The listing builds one solid part. Answer for the finished solid, in the listing's coordinates (mm). A direction names the side the tool comes from. Round coordinates to 2 decimals unless told otherwise and drop trailing zeros. Write each loop counter-clockwise with the first axis right and the second up, starting at its lowest first coordinate (ties: lowest second). Pieces come first, ordered by that corner, then holes.
Item 1: Find section B-B on x = 5. Give the vertices of the cut face in (y, z).
Item 2: Find section A-A on z = 5. Give the vertices of the cut face in (x, y), then the cut area to 3 significant figures.
Item 3: Find section D-D on z = 70. Give the vertices of the cut face in (x, y), then the cut area to 3 significant figures.
Item 4: A tool of negligible diameter and unlimited length cuts with its end or side. For faces 4 (the face through (0.5, 5.1, 80)), 5 (the face through (1, 5, 41)), from which of +Z, -Z, +X, -X, +Y, -Y can it reach the whole face along a straight path? Write none if from no direction.
Item 5: For a pull along Z with two mould halves and no side action, classify faces 1 (the face through (10, 5, 41)), 2 (the face through (9.507, 5.481, 76.526)), 3 (the face through (0.5, 5.1, 0)) as +Z half, -Z half, draft (parallel to the pull), parting line (faces both ways), or undercut.
Item 6: Find the intervals of material crossed by probe 1 along Z at (x, y) = (5, 0.35); probe 2 along X at (y, z) = (5.75, 23.5); probe 3 along X at (y, z) = (0.7, 15), in increasing order.
Item 7: Find section C-C on y = 2.5. Give the vertices of the cut face in (x, z), then the cut area to 3 significant figures.
```python
from build123d import *

# Parameters (mm, degrees)
SKETCH_1_W          = 10
SKETCH_1_H          = 10
SKETCH_1_W_2        = 8
SKETCH_1_H_2        = 8
EXTRUDE_1_DEPTH     = 40
SKETCH_2_R          = 1.6
CUT_EXTRUDE_1_DEPTH = 11
SKETCH_3_R          = 1.6
CUT_EXTRUDE_2_DEPTH = 11


with BuildPart() as part:
    # ｽｹｯﾁ1 → ﾎﾞｽ - 押し出し1 (new body)
    with BuildSketch(Plane.XY):
        with Locations((5, 5)):
            Rectangle(SKETCH_1_W, SKETCH_1_H)
        with Locations((5, 5)):
            Rectangle(SKETCH_1_W_2, SKETCH_1_H_2, mode=Mode.SUBTRACT)
    extrude(amount=EXTRUDE_1_DEPTH)

    # ｽｹｯﾁ2 → ｶｯﾄ - 押し出し1 (cut, through all)
    with BuildSketch(Plane(origin=(10, 0, 0), x_dir=(0, 0, -1), z_dir=(1, 0, 0))):
        with Locations((-5, 5)):
            Circle(SKETCH_2_R)
    extrude(amount=-CUT_EXTRUDE_1_DEPTH, mode=Mode.SUBTRACT)

    # ｽｹｯﾁ3 → ｶｯﾄ - 押し出し2 (cut, through all)
    with BuildSketch(Plane(origin=(0, 10, 0), x_dir=(1, 0, 0), z_dir=(0, 1, 0))):
        with Locations((5, -15)):
            Circle(SKETCH_3_R)
    extrude(amount=-CUT_EXTRUDE_2_DEPTH, mode=Mode.SUBTRACT)

    # ﾐﾗｰ1: part across plane


with BuildPart() as part_1:
    add(part.part)
    add(part.part.mirror(Plane(origin=(0, 0, 40), x_dir=(1, 0, 0), z_dir=(0, 0, -1))))


solid = part_1.part
```
Check values:
1. outline: (0, 0) - (1, 0) - (1, 13.4) - (0, 13.4) - close; (0, 16.6) - (1, 16.6) - (1, 63.4) - (0, 63.4) - close; (0, 66.6) - (1, 66.6) - (1, 80) - (0, 80) - close; (9, 0) - (10, 0) - (10, 13.4) - (9, 13.4) - close; (9, 16.6) - (10, 16.6) - (10, 63.4) - (9, 63.4) - close; (9, 66.6) - (10, 66.6) - (10, 80) - (9, 80) - close
2. outline: (0, 0) - (10, 0) - (10, 3.4) - (9, 3.4) - (9, 1) - (1, 1) - (1, 3.4) - (0, 3.4) - close; (0, 6.6) - (1, 6.6) - (1, 9) - (9, 9) - (9, 6.6) - (10, 6.6) - (10, 10) - (0, 10) - close
2. area: 29.6 mm2
3. outline: (0, 0) - (10, 0) - (10, 10) - (0, 10) - close; hole (1, 1) - (9, 1) - (9, 9) - (1, 9) - close
3. area: 36.0 mm2
4. face 4: +Z, +X, -X, +Y, -Y
4. face 5: +Z, -Z
5. face 1: draft
5. face 2: undercut
5. face 3: -Z half
6. probe 1: z = 0 to 13.4, 16.6 to 63.4, 66.6 to 80
6. probe 2: x = 0 to 1, 9 to 10
6. probe 3: x = 0 to 3.4, 6.6 to 10
7. outline: (0, 0) - (1, 0) - (1, 80) - (0, 80) - close; (9, 0) - (10, 0) - (10, 80) - (9, 80) - close
7. area: 160 mm2
